from build123d import *

# Parameters (mm, degrees)
F3_R     = 5
F4_DEPTH = 2.5
F5_DEPTH = 2.5


with BuildPart() as f2:
    # F2: sweep along a path in F1
    with BuildLine(Plane.XZ) as f2_path:
        Line((0, 0), (-80, 0))
        ThreePointArc((-80, 0), (-101.2132034356, -8.7867965644), (-110, -30))
        Line((-110, -30), (-110, -110))
        ThreePointArc((-110, -110), (-101.2132034356, -131.2132034356), (-80, -140))
        Line((-80, -140), (0, -140))
    # F0 (on Right) → F2 (sweep)
    with BuildSketch(Plane.YZ):
        with BuildLine():
            Line((10, 20), (0, 20))
            Line((0, 20), (-10, 20))
            Line((-10, 20), (-10, 15))
            Line((-10, 15), (-5.5, 15))
            ThreePointArc((-5.5, 15), (-3.3786796564, 14.1213203436), (-2.5, 12))
            Line((-2.5, 12), (-2.5, 0))
            Line((-2.5, 0), (-2.5, -12))
            ThreePointArc((-2.5, -12), (-3.3786796564, -14.1213203436), (-5.5, -15))
            Line((-5.5, -15), (-10, -15))
            Line((-10, -15), (-10, -20))
            Line((-10, -20), (0, -20))
            Line((0, -20), (10, -20))
            Line((10, -20), (10, -15))
            Line((10, -15), (5.5, -15))
            ThreePointArc((5.5, -15), (3.3786796564, -14.1213203436), (2.5, -12))
            Line((2.5, -12), (2.5, 0))
            Line((2.5, 0), (2.5, 12))
            ThreePointArc((2.5, 12), (3.3786796564, 14.1213203436), (5.5, 15))
            Line((5.5, 15), (10, 15))
            Line((10, 15), (10, 20))
        make_face()
    sweep(path=f2_path.line)

    # F3 (on Front) → F4 (join, symmetric)
    with BuildSketch(Plane.XZ):
        with BuildLine():
            Line((-70, 20), (0, 20))
            Line((0, 20), (0, 50))
            ThreePointArc((0, 50), (-13.9930064723, 59.3289627376), (-30.1564242691, 54.6837823298))
            Line((-30.1564242691, 54.6837823298), (-70, 20))
        make_face()
        with Locations((-20, 47.5595779717)):
            Circle(F3_R, mode=Mode.SUBTRACT)
    extrude(amount=F4_DEPTH, both=True)

    # F3 (on Front) → F5 (join, symmetric)
    with BuildSketch(Plane.XZ):
        with BuildLine():
            Line((-70, 20), (0, 20))
            Line((0, 20), (0, 50))
            ThreePointArc((0, 50), (-13.9930064723, 59.3289627376), (-30.1564242691, 54.6837823298))
            Line((-30.1564242691, 54.6837823298), (-70, 20))
        make_face()
        with Locations((-20, 47.5595779717)):
            Circle(F3_R, mode=Mode.SUBTRACT)
        with BuildLine():
            Line((-0.4077370701, -160), (-70.4077370701, -160))
            Line((-70.4077370701, -160), (-30.6394707567, -194.618225577))
            ThreePointArc((-30.6394707567, -194.618225577), (-14.4500845673, -199.3365631453), (-0.4077370701, -190))
            Line((-0.4077370701, -190), (-0.4077370701, -160))
        make_face()
        with Locations((-20.4077370701, -190.2831075506)):
            Circle(F3_R, mode=Mode.SUBTRACT)
    extrude(amount=F5_DEPTH, both=True)


solid = f2.part
Read the model definition and answer for the solid it produces. Units are mm, in the model's axes. A direction names the side the tool comes from. Coordinates: 2 decimals unless noted, no trailing zeros. Loops run counter-clockwise (first coordinate to the right, second up) from the corner with the lowest first, then second, coordinate; pieces in that order, holes last. Notation, with made-up numbers: (87, 33) - (126, 33) arc R12 ccw to (126, 45) - close; hole circle Ø7 at (-23.75, -28). An arc over 180 degrees is marked (long way). Answer in a Markdown table with one row per item.
Q1. The mould has two halves that part along X. Classify faces 5 (the flat face through (-0.408, 0, -175)), 6 (the flat face through (-128, -10, -70)), 7 (the cylindrical face through (-21.059, 0.035, -185.326)): pulls with the +X half, pulls with the -X half, needs draft (parallel to the pull), parting line crosses it, or undercut.
Here are the results:
| item | result |
|---|---|
| face 5 | pulls with the +X half |
| face 6 | needs draft |
| face 7 | undercut |
Q2. For faces 1 (the flat face through (-41, 8, 15)), 2 (the flat face through (-41, -8, 15)), 3 (the cylindrical face through (-90.72, 7.72, -120.49)), 4 (the cylindrical face through (-90.72, -7.78, -120.49)), determine the directions among +Z, -Z, +X, -X, +Y, -Y from which every point of the face is accessible in a straight line to the end or side of a thin tool.
Here are the results:
| item | result |
|---|---|
| face 1 | +X, +Y |
| face 2 | +X, -Y |
| face 3 | +Y |
| face 4 | -Y |
Q3. Straight lines are drawn through the part: line 1 along Z through (x, y) = (-77.5, -7.75); line 2 along Z through (x, y) = (-20, -0.5); line 3 along X through (y, z) = (-1.5, -102). For each, find the intervals that lie inside material, in ascending order. Write a range as [from, to].
Here are the results:
| item | result |
|---|---|
| line 1 | z = [-160, -155], [-125, -120], [-20, -15], [15, 20] |
| line 2 | z = [-199.41, -195.27], [-185.3, -120], [-20, 42.56], [52.56, 59.35] |
| line 3 | x = [-130, -90] |
Q4. Given P1, Ø6, axis at x = -38, z = -6.5, coming from the -Y side; P2, Ø10, axis at x = -54, y = -1, coming from the -Z side; P3, Ø11.5, axis at x = -20, z = 47.56, coming from the +Y side, each flat-ended and moving along its own axis, determine where each tip first touches the part or whether it passes through.
Here are the results:
| item | result |
|---|---|
| P1 | stops at y = -2.5 |
| P2 | stops at z = -178.64 |
| P3 | stops at y = 2.5 |
Q5. Find section C-C on x = -20. Count the separate pieces of the cut face and the enclosed holes in it, plus the area to 3 significant figures.
Here are the results:
| item | result |
|---|---|
| separate pieces | 4 |
| enclosed holes | 0 |
| area | 1,010 mm^2 |
Q6. Find section B-B on z = -53.5. Write down the section's boundary in (x, y), plus the area to 3 significant figures.
Here are the results:
| item | result |
|---|---|
| outline | (-130, -10) - (-125, -10) - (-125, -5.5) arc R3 cw to (-122, -2.5) - (-98, -2.5) arc R3 cw to (-95, -5.5) - (-95, -10) - (-90, -10) - (-90, 10) - (-95, 10) - (-95, 5.5) arc R3 cw to (-98, 2.5) - (-122, 2.5) arc R3 cw to (-125, 5.5) - (-125, 10) - (-130, 10) - close |
| area | 358 mm^2 |
